Check sheet for the modelled part. Datum: model origin and axes. Units: mm. Give positions to 0.01 mm unless a question says otherwise; leave off trailing zeros. Order: outer loops, then holes, each group sorted by start corner. A loop starts at its lowest first (then second) coordinate and runs counter-clockwise, first axis right, second up.
from build123d import *

# Parameters (mm, degrees)
F1_DEPTH = 6.35
F2_D     = 4.826
F3_D     = 3.81
F5_DEPTH = 25.4


# Not quite as in the source:
# - a feature names something its author has since deleted; it is built from what else it names


with BuildPart() as f1:
    # F0 (on Right) → F1 (new body)
    with BuildSketch(Plane.YZ):
        Polygon((274.6375, -12.7), (274.6375, 0), (274.6375, 53.8988), (0, 53.8988), (0, 0), (0, -12.7), align=None)
    extrude(amount=F1_DEPTH)

    # F2 (through all)
    with Locations(Plane(origin=(0, 0, 0), x_dir=(0, 1, 0), z_dir=(-1, 0, 0))):
        with Locations((4.7625, -40.4241), (4.7625, -26.9494), (4.7625, -13.4747)):
            Hole(F2_D / 2)

    # F3 (through all)
    with Locations(Plane(origin=(0, 0, 0), x_dir=(0, 1, 0), z_dir=(-1, 0, 0))):
        with Locations((271.4625, -40.4241), (271.4625, -26.9494), (271.4625, -13.4747)):
            Hole(F3_D / 2)

    # F4 (on face) → F5 (cut)
    with BuildSketch(Plane.YZ.offset(6.35)):
        Polygon((0, 53.8988), (0, 49.6316), (25.4, 49.6316), (41.275, 33.7566), (233.3625, 33.7566), (249.2375, 49.6316), (274.6375, 49.6316), (274.6375, 53.8988), align=None)
    extrude(amount=-F5_DEPTH, mode=Mode.SUBTRACT)


solid = f1.part
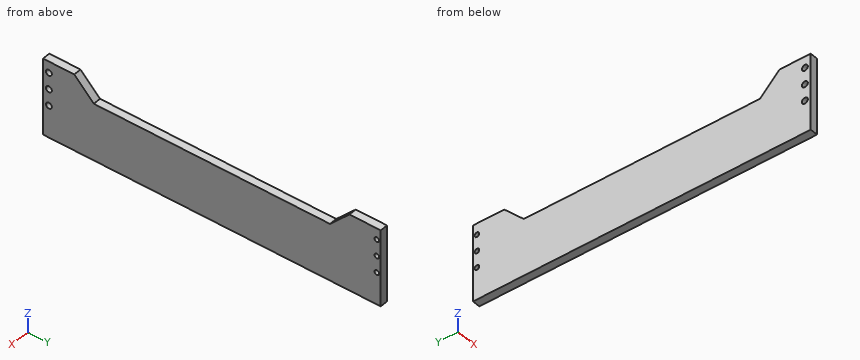
1) Section check B-B, the plane y = 226. Record the cut outline in (x, z).
Recorded:
outline: (0, -12.7) - (6.35, -12.7) - (6.35, 33.76) - (0, 33.76) - close
2) Section check A-A, the plane x = 2.25. Record the cut outline in (y, z) (1 decimal).
Recorded:
outline: (0, -12.7) - (274.6, -12.7) - (274.6, 49.6) - (249.2, 49.6) - (233.4, 33.8) - (41.3, 33.8) - (25.4, 49.6) - (0, 49.6) - close; hole circle Ø4.8 at (4.8, 13.5); hole circle Ø4.8 at (4.8, 26.9); hole circle Ø4.8 at (4.8, 40.4); hole circle Ø3.8 at (271.5, 13.5); hole circle Ø3.8 at (271.5, 26.9); hole circle Ø3.8 at (271.5, 40.4)
3) Depth check by flat-ended pin: pin 1 Ø5.5 at (y, z) = (4.76, 40.42) entering from -X; pin 2 Ø1.5 at (x, y) = (1.5, 98.5) entering from +Z; pin 3 Ø4.5 at (y, z) = (4.76, 26.95) entering from +X. Enter the tip coordinate at first touch or a pass-through.
Recorded:
pin 1: stops at x = 0
pin 2: stops at z = 33.76
pin 3: passes through
4) Material ranges on L1, parallel to Y at x = 3.5, z = 27; L2, parallel to Y at x = 0.75, z = 12; L3, parallel to Z at x = 0.5, y = 228, recorded low to high.
Recorded:
L1: y = 0 to 2.35, 7.17 to 269.56, 273.37 to 274.64
L2: y = 0 to 2.85, 6.67 to 270.26, 272.67 to 274.64
L3: z = -12.7 to 33.76
